Study the drawing (mm; zero at the part's minimum x, y, z) and answer. Round coordinates to 2 decimals unless told otherwise and drop trailing zeros. Loops run counter-clockwise (first coordinate to the right, second up) from the corner with the lowest first, then second, coordinate; pieces in that order, holes last. Notation, with made-up numbers: (81.5, 51.5) - (119.5, 51.5) arc R29 ccw to (119.5, 71.5) - close; hole circle Ø9 at (18, 5). An arc over 180 degrees is marked (long way). One line per item, written item: value.
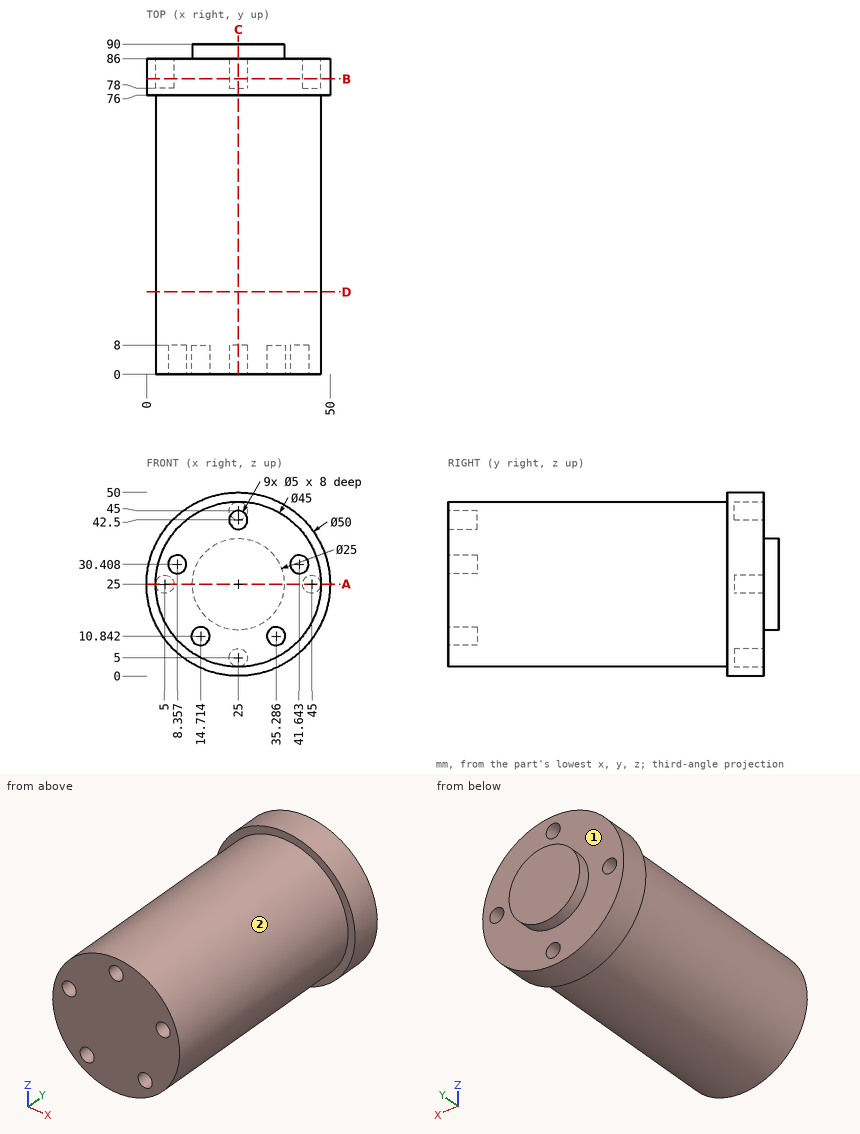
1) For a pull along X with two mould halves and no side action, classify the marked faces 1 and 2 as released by +X, released by -X, zero draft, split by the parting line, or undercut.
Final values:
face 1: zero draft
face 2: split by the parting line
2) A cutting plane is placed at A-A on z = 25. Give the vertices of the cut face in (x, y), and give its area (3 significant figures).
Final values:
outline: (0, 76) - (2.5, 76) - (2.5, 0) - (47.5, 0) - (47.5, 76) - (50, 76) - (50, 86) - (47.5, 86) - (47.5, 78) - (42.5, 78) - (42.5, 86) - (37.5, 86) - (37.5, 90) - (12.5, 90) - (12.5, 86) - (7.5, 86) - (7.5, 78) - (2.5, 78) - (2.5, 86) - (0, 86) - close
area: 3,940 mm2
3) Consider L1, parallel to X at y = 5.5, z = 42.5 (1 decimal); L2, parallel to Y at x = 39, z = 41; L3, parallel to Z at x = 45, y = 83. Determine where each line is inside the solid, lowest interval first.
Final values:
L1: 10.9 to 22.5, 27.5 to 39.1
L2: 0 to 86
L3: 10 to 22.5, 27.5 to 40
4) A cutting plane is placed at D-D on y = 22.5. Give the vertices of the cut face in (x, z).
Final values:
outline: circle Ø45 at (25, 25)
5) Each of these flat-tipped pins is pushed along its axis until it touches: pin 1 Ø2.5 at (x, z) = (25.5, 46) entering from +Y; pin 2 Ø1.5 at (x, z) = (35.5, 30) entering from -Y; pin 3 Ø1 at (y, z) = (46, 26.5) entering from +X; pin 4 Ø12 at (y, z) = (49.5, 10) entering from +X. Where does it stop, or does it pass through?
Final values:
pin 1: y = 78
pin 2: y = 0
pin 3: x = 47.48
pin 4: x = 45.62
6) A cutting plane is placed at C-C on x = 25. Give the vertices of the cut face in (y, z).
Final values:
outline: (0, 2.5) - (76, 2.5) - (76, 0) - (86, 0) - (86, 2.5) - (78, 2.5) - (78, 7.5) - (86, 7.5) - (86, 12.5) - (90, 12.5) - (90, 37.5) - (86, 37.5) - (86, 42.5) - (78, 42.5) - (78, 47.5) - (86, 47.5) - (86, 50) - (76, 50) - (76, 47.5) - (0, 47.5) - (0, 45) - (8, 45) - (8, 40) - (0, 40) - close
7) A cutting plane is placed at B-B on y = 80.5. Give the vertices of the cut face in (x, z), and give its area (4 significant figures).
Final values:
outline: circle Ø50 at (25, 25); hole circle Ø5 at (5, 25); hole circle Ø5 at (25, 5); hole circle Ø5 at (25, 45); hole circle Ø5 at (45, 25)
area: 1,885 mm2
